Model file for the job. Use its own axes, mm. A direction names the side the tool comes from. Round coordinates to 2 decimals unless told otherwise and drop trailing zeros. Loops run counter-clockwise (first coordinate to the right, second up) from the corner with the lowest first, then second, coordinate; pieces in that order, holes last. Notation, with made-up numbers: M -35.75,31 L 23.25,31 A23 ccw 23.25,42 Z; hole C 67.25,-15.75 d3. An arc over 180 degrees is marked long. Use a Markdown table: item, result. Add a question column.
Item 1: Saw through at A-A on z = 0. Write the cut outline in (x, y) (3 decimals), then the cut area to 3 significant figures.
Item 2: Wall check: L1, parallel to X at y = -2.5, z = 2 (3 decimals); L2, parallel to Y at x = -1.5, z = 0. Give the ranges that are in metal, low to high. Write a range as from..to.
Item 3: Tool access for faces 1 (the cylindrical face through (3.01, 1.27, 1.99)), 2 (the flat face through (9.525, 0, 0)): list every direction of +Z, -Z, +X, -X, +Y, -Y with a clear straight run to the whole face (end or side of a thin tool).
Item 4: Pin check, flat tips, straight feed: P1, Ø3, axis at x = 3, z = -1.5, coming from the -Y side; P2, Ø1, axis at x = -3.5, y = -1.5, coming from the +Z side; P3, Ø5, axis at x = -1.5, z = 2.5, coming from the -Y side. Stop position of each tip, or through.
Item 5: Saw through at D-D on x = -8. Write the cut outline in (y, z) (3 decimals).
Item 6: Saw through at C-C on x = 4.75. Write the cut outline in (y, z), then the cut area to 3 significant figures.
```python
from build123d import *

# Parameters (mm, degrees)
F0_R     = 2.3622
F1_DEPTH = 9.525
F2_R     = 4.445
F2_R_2   = 2.3622
F3_DEPTH = 6.35
F4_SIZE  = 0.508


with BuildPart() as f1:
    # F0 (on Right) → F1 (new body, symmetric)
    with BuildSketch(Plane.YZ):
        Circle(F0_R)
    extrude(amount=F1_DEPTH, both=True)

    # F2 (on face) → F3 (join)
    with BuildSketch(Plane(origin=(-9.525, 0, 0), x_dir=(0, -1, 0), z_dir=(-1, 0, 0))):
        Circle(F2_R)
        Circle(F2_R_2, mode=Mode.SUBTRACT)
    extrude(amount=-F3_DEPTH)

    # F4
    f4_edges = [f1.edges().sort_by_distance(p)[0] for p in [
        (9.525, -2.3622, 0),
    ]]
    chamfer(f4_edges, length=F4_SIZE)


solid = f1.part
```
Entries:
| question | item | result |
|---|---|---|
| 1 | outline | M -9.525,-4.445 L -3.175,-4.445 L -3.175,-2.362 L 9.017,-2.362 L 9.525,-1.854 L 9.525,1.854 L 9.017,2.362 L -3.175,2.362 L -3.175,4.445 L -9.525,4.445 Z |
| 1 | area | 116 mm2 |
| 2 | L1 | -9.525..-3.175 |
| 2 | L2 | -2.36..2.36 |
| 3 | face 1 | +X |
| 3 | face 2 | +Z, -Z, +X, +Y, -Y |
| 4 | P1 | y = -2.36 |
| 4 | P2 | z = 4.33 |
| 4 | P3 | y = -4.4 |
| 5 | outline | C 0,0 d8.89 |
| 6 | outline | C 0,0 d4.72 |
| 6 | area | 17.5 mm2 |
